For this review, use the dimensioned drawing (mm, ordinates from the lowest corner) and the shaded views. Give positions to 0.01 mm unless a question says otherwise; leave off trailing zeros. Loops run counter-clockwise (first coordinate to the right, second up) from the corner with the lowest first, then second, coordinate; pieces in that order, holes last. Notation, with made-up numbers: (86.5, 80) - (96.5, 80) arc R19 ccw to (96.5, 110) - close; hole circle Ø5 at (-28, 75). An arc over 180 degrees is marked (long way). Write each question's results on one line, items separated by ' | '.
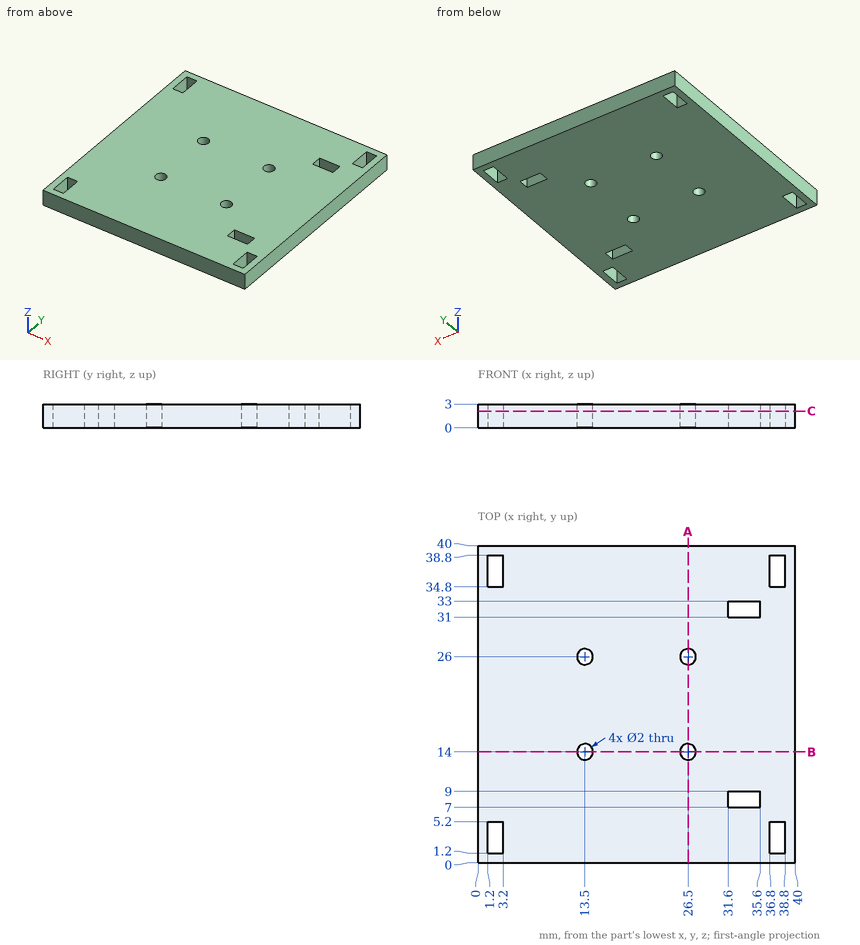
Item 1: Wall thickness on probe 1 along Y at (x, z) = (26.5, 1.8); probe 2 along Y at (x, z) = (34, 2.75); probe 3 along X at (y, z) = (3.5, 2.75): over which ranges is each line inside the solid? List them lowest first.
Output values:
probe 1: y = 0 to 13, 15 to 25, 27 to 40 | probe 2: y = 0 to 7, 9 to 31, 33 to 40 | probe 3: x = 0 to 1.2, 3.2 to 36.8, 38.8 to 40
Item 2: We need section B-B on y = 14. Give the boundary of the cut face in (x, z), then the cut area to 3 significant figures.
Output values:
outline: (0, 0) - (12.5, 0) - (12.5, 3) - (0, 3) - close; (14.5, 0) - (25.5, 0) - (25.5, 3) - (14.5, 3) - close; (27.5, 0) - (40, 0) - (40, 3) - (27.5, 3) - close | area: 108 mm²
Item 3: We need section C-C on z = 2.1. Give the number of separate pieces and of enclosed holes in the cut face, then the cut area to 3 significant figures.
Output values:
separate pieces: 1 | enclosed holes: 10 | area: 1,540 mm²
Item 4: We need section A-A on x = 26.5. Give the boundary of the cut face in (y, z), then the cut area to 3 significant figures.
Output values:
outline: (0, 0) - (13, 0) - (13, 3) - (0, 3) - close; (15, 0) - (25, 0) - (25, 3) - (15, 3) - close; (27, 0) - (40, 0) - (40, 3) - (27, 3) - close | area: 108 mm²
